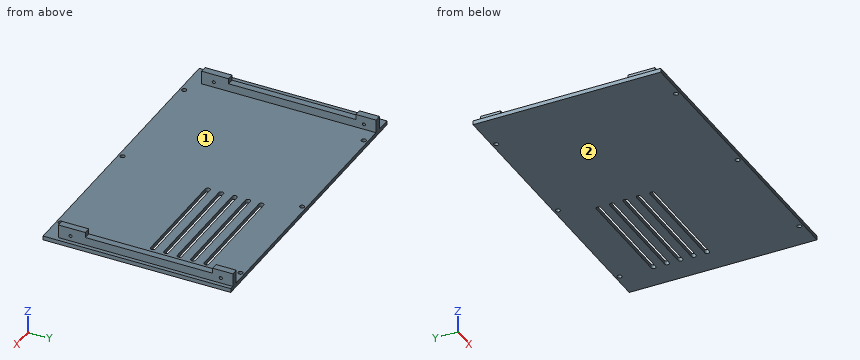
```python
from build123d import *

# Parameters (mm, degrees)
SKETCH_W     = 228
SKETCH_H     = 140
SKETCH_R     = 1.75
PAD_DEPTH    = 3
SKETCH001_W  = 5
SKETCH001_H  = 130
PAD001_DEPTH = 10
SKETCH002_R  = 1.15
SKETCH002_W  = 95
SKETCH002_H  = 4
POCKET_DEPTH = 225


with BuildPart() as part:
    # Sketch → Pad (new body)
    with BuildSketch(Plane.XY):
        with Locations((-4, 0)):
            Rectangle(SKETCH_W, SKETCH_H)
        with Locations((-90, 67)):
            Circle(SKETCH_R, mode=Mode.SUBTRACT)
        with Locations((0, 67)):
            Circle(SKETCH_R, mode=Mode.SUBTRACT)
        with Locations((90, 67)):
            Circle(SKETCH_R, mode=Mode.SUBTRACT)
        with Locations((-90, -67)):
            Circle(SKETCH_R, mode=Mode.SUBTRACT)
        with Locations((0, -67)):
            Circle(SKETCH_R, mode=Mode.SUBTRACT)
        with Locations((90, -67)):
            Circle(SKETCH_R, mode=Mode.SUBTRACT)
        with BuildLine():
            ThreePointArc((10.059248, 43.499956), (8.309248, 41.749956), (10.059248, 39.999956))
            Line((10.059248, 39.999956), (90.059248, 39.999956))
            ThreePointArc((90.059248, 39.999956), (91.809248, 41.749956), (90.059248, 43.499956))
            Line((10.059248, 43.499956), (90.059248, 43.499956))
        make_face(mode=Mode.SUBTRACT)
        with BuildLine():
            ThreePointArc((10.044436, 33.499967), (8.294436, 31.749967), (10.044436, 29.999967))
            Line((10.044436, 29.999967), (90.044436, 29.999967))
            ThreePointArc((90.044436, 29.999967), (91.794436, 31.749967), (90.044436, 33.499967))
            Line((10.044436, 33.499967), (90.044436, 33.499967))
        make_face(mode=Mode.SUBTRACT)
        with BuildLine():
            ThreePointArc((10.029624, 23.499978), (8.279624, 21.749978), (10.029624, 19.999978))
            Line((10.029624, 19.999978), (90.029624, 19.999978))
            ThreePointArc((90.029624, 19.999978), (91.779624, 21.749978), (90.029624, 23.499978))
            Line((10.029624, 23.499978), (90.029624, 23.499978))
        make_face(mode=Mode.SUBTRACT)
        with BuildLine():
            ThreePointArc((10.014812, 13.499989), (8.264812, 11.749989), (10.014812, 9.999989))
            Line((10.014812, 9.999989), (90.014812, 9.999989))
            ThreePointArc((90.014812, 9.999989), (91.764812, 11.749989), (90.014812, 13.499989))
            Line((10.014812, 13.499989), (90.014812, 13.499989))
        make_face(mode=Mode.SUBTRACT)
        with BuildLine():
            ThreePointArc((10, 3.5), (8.25, 1.75), (10, 0))
            Line((10, 0), (90, 0))
            ThreePointArc((90, 0), (91.75, 1.75), (90, 3.5))
            Line((10, 3.5), (90, 3.5))
        make_face(mode=Mode.SUBTRACT)
    extrude(amount=PAD_DEPTH)

    # Sketch001 → Pad001 (join)
    with BuildSketch(Plane.XY.offset(3)):
        with Locations((104.5, 5)):
            Rectangle(SKETCH001_W, SKETCH001_H)
        with Locations((-104.5, 5)):
            Rectangle(SKETCH001_W, SKETCH001_H)
    extrude(amount=PAD001_DEPTH)

    # Sketch002 → Pocket (cut)
    with BuildSketch(Plane.YZ.offset(107)):
        with Locations((-51, 7)):
            Circle(SKETCH002_R)
        with Locations((61, 7)):
            Circle(SKETCH002_R)
        with Locations((7.5, 11)):
            Rectangle(SKETCH002_W, SKETCH002_H)
    extrude(amount=-POCKET_DEPTH, mode=Mode.SUBTRACT)


solid = part.part
```
Verification items for the finished model (mm, model axes). Face numbers are marked on the shaded views. Round coordinates to 2 decimals unless told otherwise and drop trailing zeros. Write each loop counter-clockwise with the first axis right and the second up, starting at its lowest first coordinate (ties: lowest second). Pieces come first, ordered by that corner, then holes.
1. Draft check along X on the marked faces 1 and 2. Enter one of: +X half, -X half, draft (parallel to the pull), parting line (faces both ways), or undercut.
2. Gauge pin test, flat ends, axial feed: P1, Ø5.5, axis at x = 103.5, z = 6.5, coming from the -Y side; P2, Ø3.5, axis at y = 61, z = 7, coming from the +X side; P3, Ø3, axis at y = 27.5, z = 8.5, coming from the -X side; P4, Ø10, axis at x = 27.5, y = 0, coming from the -Z side. Record the tip position at first contact, or that the pin passes through.
3. Section check C-C on x = -5. Enter the section's corners in (y, z).
4. Section check A-A on x = 78. Enter the section's corners in (y, z).
5. Section check B-B on y = -9. Enter the section's corners in (x, z), plus the area to 3 significant figures.
6. Scan lines: L1, parallel to Y at x = 0, z = 1.95; L2, parallel to X at y = -67, z = 2.25; L3, parallel to Z at x = -105, y = 61. Record each from-to range of solid material in increasing order.
Answer:
1. face 1: undercut
1. face 2: draft
2. P1: stops at y = -60
2. P2: stops at x = 107
2. P3: stops at x = -107
2. P4: stops at z = 0
3. outline: (-70, 0) - (70, 0) - (70, 3) - (-70, 3) - close
4. outline: (-70, 0) - (0, 0) - (0, 3) - (-70, 3) - close; (3.5, 0) - (10, 0) - (10, 3) - (3.5, 3) - close; (13.5, 0) - (20, 0) - (20, 3) - (13.5, 3) - close; (23.5, 0) - (30, 0) - (30, 3) - (23.5, 3) - close; (33.5, 0) - (40, 0) - (40, 3) - (33.5, 3) - close; (43.5, 0) - (70, 0) - (70, 3) - (43.5, 3) - close
5. outline: (-118, 0) - (110, 0) - (110, 3) - (107, 3) - (107, 9) - (102, 9) - (102, 3) - (-102, 3) - (-102, 9) - (-107, 9) - (-107, 3) - (-118, 3) - close
5. area: 744 mm2
6. L1: y = -70 to -68.75, -65.25 to 65.25, 68.75 to 70
6. L2: x = -118 to -91.75, -88.25 to -1.75, 1.75 to 88.25, 91.75 to 110
6. L3: z = 0 to 5.85, 8.15 to 13
